```python
from build123d import *

# Parameters (mm, degrees)
SKETCH1_W           = 25
SKETCH1_H           = 5
BOSS_EXTRUDE1_DEPTH = 35
BOSS_EXTRUDE2_DEPTH = 3


with BuildPart() as part:
    # Sketch1 → Boss-Extrude1 (new body)
    with BuildSketch(Plane.XY):
        with Locations((12.5, -2.5)):
            Rectangle(SKETCH1_W, SKETCH1_H)
    extrude(amount=BOSS_EXTRUDE1_DEPTH)

    # Sketch2 → Boss-Extrude2 (add)
    with BuildSketch(Plane.XY.offset(35)):
        with BuildLine():
            Line((10.5, -1.75), (14.5, -1.75))
            ThreePointArc((14.5, -1.75), (15.25, -2.5), (14.5, -3.25))
            Line((14.5, -3.25), (10.5, -3.25))
            ThreePointArc((10.5, -3.25), (9.75, -2.5), (10.5, -1.75))
        make_face()
    extrude(amount=BOSS_EXTRUDE2_DEPTH)


solid = part.part
```
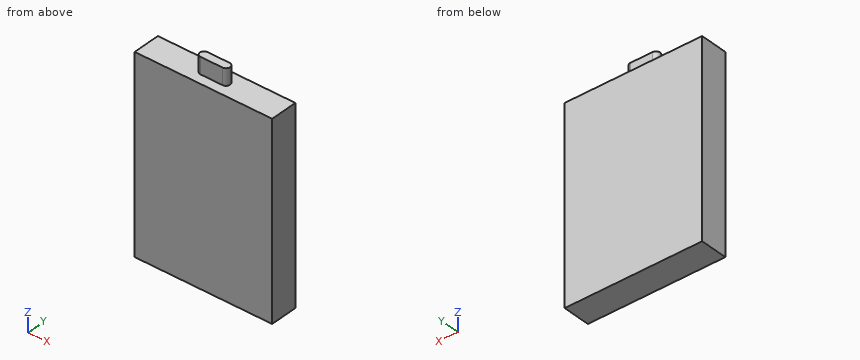
Check sheet for the modelled part. Datum: model origin and axes. Units: mm. Round coordinates to 2 decimals unless told otherwise and drop trailing zeros. Order: outer loops, then holes, each group sorted by start corner. A loop starts at its lowest first (then second) coordinate and runs counter-clockwise, first axis right, second up.
1) Go/stop test with flat-tipped pins: pin 1 Ø2.5 at (x, z) = (12.5, 36.5) entering from +Y; pin 2 Ø1.5 at (x, z) = (13.5, 36) entering from -Y. Record where each tip stops, or that it passes through.
2) Section check A-A (y = -2.5). Record the boundary of the cut face in (x, z).
3) Section check B-B (x = 23.75). Record the boundary of the cut face in (y, z).
4) Scan line: line 1 (Z direction, x = 1, y = -3.55). Record every from-to range of solid material in increasing order.
Result:
1. pin 1: stops at y = -1.75
1. pin 2: stops at y = -3.25
2. outline: (0, 0) - (25, 0) - (25, 35) - (15.25, 35) - (15.25, 38) - (9.75, 38) - (9.75, 35) - (0, 35) - close
3. outline: (-5, 0) - (0, 0) - (0, 35) - (-5, 35) - close
4. line 1: z = 0 to 35
